```python
from build123d import *

# Parameters (mm, degrees)
F0_R     = 1.25
F1_DEPTH = 2.4
F2_SIZE  = 0.2


with BuildPart() as f1:
    # F0 (on Top) → F1 (new body)
    with BuildSketch(Plane.XY):
        Polygon((1.587713, 2.75), (-1.587713, 2.75), (-3.175426, 0), (-1.587713, -2.75), (1.587713, -2.75), (3.175426, 0), align=None)
        Circle(F0_R, mode=Mode.SUBTRACT)
    extrude(amount=F1_DEPTH)

    # F2
    f2_edges = [f1.edges().sort_by_distance(p)[0] for p in [
        (-1.25, 0, 2.4),
        (-1.25, 0, 0),
    ]]
    chamfer(f2_edges, length=F2_SIZE)

    # F3 (on Front) → F4 (revolve, cut)
    with BuildSketch(Plane.XZ):
        Polygon((3.375426, 0.625426), (2.75, 0), (3.738599, 0), (3.738599, 2.737111), (2.75, 2.737111), (2.75, 2.4), (3.375426, 1.774574), align=None)
    revolve(axis=Axis((0, 0, 1.849946), (0, 0, 1)), mode=Mode.SUBTRACT)


solid = f1.part
```
The model under review builds one solid part; all positions refer to its coordinate system, in mm. Round coordinates to 2 decimals unless told otherwise and drop trailing zeros. Order: outer loops, then holes, each group sorted by start corner. A loop starts at its lowest first (then second) coordinate and runs counter-clockwise, first axis right, second up. Notation, with made-up numbers: M 24,16.5 L 53,16.5 A15 ccw 53,35.5 Z; hole C 62.25,57 d1. An arc over 180 degrees is marked long. Use a Markdown table: item, result.
1) Consider section A-A (z = 0.65). Write out the cut boundary in (x, y).
Report:
| item | result |
|---|---|
| outline | M -3.18,0 L -1.59,-2.75 L 1.59,-2.75 L 3.18,0 L 1.59,2.75 L -1.59,2.75 Z; hole C 0,0 d2.5 |
2) Draft analysis for pull direction X (two halves, no side actions). For faces 1 (the face through (1.448, 2.495, 2.265)), 2 (the face through (1.2, -1.2, 0)), 3 (the face through (-0.27, -1.22, 1.19)), state which applies: released by +X, released by -X, zero draft, split by the parting line, or undercut.
Report:
| item | result |
|---|---|
| face 1 | released by +X |
| face 2 | zero draft |
| face 3 | undercut |
3) Wall thickness on line 1 along Y through (x, z) = (0, 0.9); line 2 along Y through (x, z) = (0.5, 0.7); line 3 along X through (y, z) = (0.7, 1.7): over which ranges is each line inside the solid? List them lowest first. Write a range as [from, to].
Report:
| item | result |
|---|---|
| line 1 | [-2.75, -1.25], [1.25, 2.75] |
| line 2 | [-2.75, -1.15], [1.15, 2.75] |
| line 3 | [-2.77, -1.04], [1.04, 2.77] |
